```python
from build123d import *

# Parameters (mm, degrees)
SKETCH_1_W          = 103.9
SKETCH_1_H          = 75.8
EXTRUDE_1_DEPTH     = 5.7
SKETCH_2_R          = 3
SKETCH_2_R_2        = 1.65
SKETCH_2_W          = 5
SKETCH_2_H          = 4
SKETCH_2_R_3        = 1.15
SKETCH_2_W_2        = 9
EXTRUDE_2_DEPTH     = 2.5
FILLET_1_R          = 1
SKETCH_3_R          = 2.5
CUT_EXTRUDE_1_DEPTH = 1
SKETCH_4_W          = 95.04
SKETCH_4_H          = 53.86
CUT_EXTRUDE_2_DEPTH = 3


with BuildPart() as part:
    # 草图1 → 凸台-拉伸1 (new body)
    with BuildSketch(Plane(origin=(0, 0, 0), x_dir=(1, 0, 0), z_dir=(0, 1, 0))):
        Rectangle(SKETCH_1_W, SKETCH_1_H)
    extrude(amount=EXTRUDE_1_DEPTH)

    # 草图2 → 凸台-拉伸2 (add)
    # profile 1 of 12: a face of its own
    with BuildSketch(Plane(origin=(0, 0, 0), x_dir=(1, 0, 0), z_dir=(0, 1, 0))):
        with BuildLine():
            ThreePointArc((-53.4, 20.95), (-54.278679656, 18.828679656), (-56.4, 17.95))
            Line((-56.4, 17.95), (-51.95, 17.95))
            Line((-51.95, 17.95), (-51.95, 23.95))
            Line((-51.95, 23.95), (-56.4, 23.95))
            ThreePointArc((-56.4, 23.95), (-54.278679656, 23.071320344), (-53.4, 20.95))
        make_face()
    # profile 2 of 12: a face of its own
    with BuildSketch(Plane(origin=(0, 0, 0), x_dir=(1, 0, 0), z_dir=(0, 1, 0))):
        with Locations((-56.4, 20.95)):
            Circle(SKETCH_2_R)
        with Locations(Location((-56.4, 20.95, 0), (0, 0, 270))):
            Circle(SKETCH_2_R_2, mode=Mode.SUBTRACT)
    # profile 3 of 12: a face of its own
    with BuildSketch(Plane(origin=(0, 0, 0), x_dir=(1, 0, 0), z_dir=(0, 1, 0))):
        with Locations((-24.55, 39.9)):
            Rectangle(SKETCH_2_W, SKETCH_2_H)
        with Locations(Location((-24.55, 39.9, 0), (0, 0, 270))):
            Circle(SKETCH_2_R_3, mode=Mode.SUBTRACT)
    # profile 4 of 12: a face of its own
    with BuildSketch(Plane(origin=(0, 0, 0), x_dir=(1, 0, 0), z_dir=(0, 1, 0))):
        with Locations((24.55, 39.9)):
            Rectangle(SKETCH_2_W, SKETCH_2_H)
        with Locations(Location((24.55, 39.9, 0), (0, 0, 270))):
            Circle(SKETCH_2_R_3, mode=Mode.SUBTRACT)
    # profile 5 of 12: a face of its own
    with BuildSketch(Plane(origin=(0, 0, 0), x_dir=(1, 0, 0), z_dir=(0, 1, 0))):
        with BuildLine():
            Line((51.95, 17.95), (56.4, 17.95))
            ThreePointArc((56.4, 17.95), (53.4, 20.95), (56.4, 23.95))
            Line((56.4, 23.95), (51.95, 23.95))
            Line((51.95, 23.95), (51.95, 17.95))
        make_face()
    # profile 6 of 12: a face of its own
    with BuildSketch(Plane(origin=(0, 0, 0), x_dir=(1, 0, 0), z_dir=(0, 1, 0))):
        with Locations((56.4, 20.95)):
            Circle(SKETCH_2_R)
        with Locations(Location((56.4, 20.95, 0), (0, 0, 270))):
            Circle(SKETCH_2_R_2, mode=Mode.SUBTRACT)
    # profile 7 of 12: a face of its own
    with BuildSketch(Plane(origin=(0, 0, 0), x_dir=(1, 0, 0), z_dir=(0, 1, 0))):
        with Locations((56.4, -20.95)):
            Circle(SKETCH_2_R)
        with Locations(Location((56.4, -20.95, 0), (0, 0, 270))):
            Circle(SKETCH_2_R_2, mode=Mode.SUBTRACT)
    # profile 8 of 12: a face of its own
    with BuildSketch(Plane(origin=(0, 0, 0), x_dir=(1, 0, 0), z_dir=(0, 1, 0))):
        with BuildLine():
            ThreePointArc((56.4, -23.95), (53.4, -20.95), (56.4, -17.95))
            Line((56.4, -17.95), (51.95, -17.95))
            Line((51.95, -17.95), (51.95, -23.95))
            Line((51.95, -23.95), (56.4, -23.95))
        make_face()
    # profile 9 of 12: a face of its own
    with BuildSketch(Plane(origin=(0, 0, 0), x_dir=(1, 0, 0), z_dir=(0, 1, 0))):
        with Locations((34.9, -39.9)):
            Rectangle(SKETCH_2_W_2, SKETCH_2_H)
        with Locations(Location((37.4, -39.9, 0), (0, 0, 270))):
            Circle(SKETCH_2_R_3, mode=Mode.SUBTRACT)
        with Locations(Location((32.4, -39.9, 0), (0, 0, 270))):
            Circle(SKETCH_2_R_3, mode=Mode.SUBTRACT)
    # profile 10 of 12: a face of its own
    with BuildSketch(Plane(origin=(0, 0, 0), x_dir=(1, 0, 0), z_dir=(0, 1, 0))):
        with Locations((-35.5, -39.9)):
            Rectangle(SKETCH_2_W, SKETCH_2_H)
        with Locations(Location((-35.5, -39.9, 0), (0, 0, 270))):
            Circle(SKETCH_2_R_3, mode=Mode.SUBTRACT)
    # profile 11 of 12: a face of its own
    with BuildSketch(Plane(origin=(0, 0, 0), x_dir=(1, 0, 0), z_dir=(0, 1, 0))):
        with Locations((-56.4, -20.95)):
            Circle(SKETCH_2_R)
        with Locations(Location((-56.4, -20.95, 0), (0, 0, 270))):
            Circle(SKETCH_2_R_2, mode=Mode.SUBTRACT)
    # profile 12 of 12: a face of its own
    with BuildSketch(Plane(origin=(0, 0, 0), x_dir=(1, 0, 0), z_dir=(0, 1, 0))):
        with BuildLine():
            ThreePointArc((-53.4, -20.95), (-54.278679656, -23.071320344), (-56.4, -23.95))
            Line((-56.4, -23.95), (-51.95, -23.95))
            Line((-51.95, -23.95), (-51.95, -17.95))
            Line((-51.95, -17.95), (-56.4, -17.95))
            ThreePointArc((-56.4, -17.95), (-54.278679656, -18.828679656), (-53.4, -20.95))
        make_face()
    extrude(amount=EXTRUDE_2_DEPTH)

    # 圆角1
    fillet_1_edges = [part.edges().sort_by_distance(p)[0] for p in [
        (-27.05, 1.25, -41.9),
        (-22.05, 1.25, -41.9),
        (22.05, 1.25, -41.9),
        (27.05, 1.25, -41.9),
        (30.4, 1.25, 41.9),
        (39.4, 1.25, 41.9),
        (-38, 1.25, 41.9),
        (-33, 1.25, 41.9),
    ]]
    fillet(fillet_1_edges, radius=FILLET_1_R)

    # 草图3 → 切除-拉伸1 (cut)
    with BuildSketch(Plane(origin=(0, 2.5, 0), x_dir=(1, 0, 0), z_dir=(0, 1, 0))):
        with Locations(Location((-56.4, -20.95, 0), (0, 0, 270))):
            Circle(SKETCH_3_R)
        with Locations(Location((-56.4, 20.95, 0), (0, 0, 270))):
            Circle(SKETCH_3_R)
        with Locations(Location((56.4, 20.95, 0), (0, 0, 270))):
            Circle(SKETCH_3_R)
        with Locations(Location((56.4, -20.95, 0), (0, 0, 270))):
            Circle(SKETCH_3_R)
    extrude(amount=-CUT_EXTRUDE_1_DEPTH, mode=Mode.SUBTRACT)

    # 草图4 → 切除-拉伸2 (cut)
    with BuildSketch(Plane(origin=(0, 5.7, 0), x_dir=(1, 0, 0), z_dir=(0, 1, 0))):
        Rectangle(SKETCH_4_W, SKETCH_4_H)
    extrude(amount=-CUT_EXTRUDE_2_DEPTH, mode=Mode.SUBTRACT)


solid = part.part
```
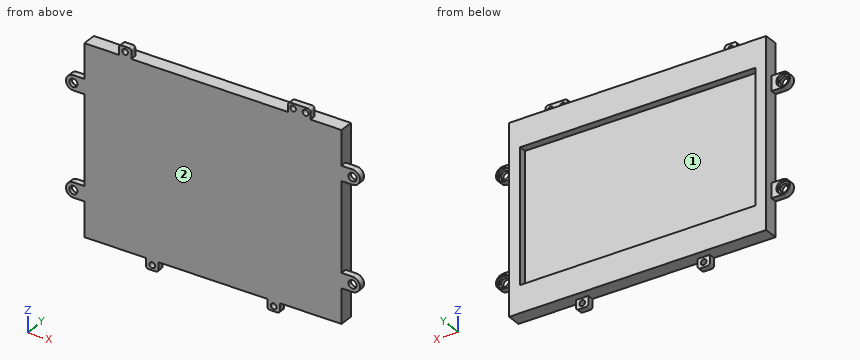
The listing builds one solid part. Answer for the finished solid, in the listing's coordinates (mm). Face numbers are marked on the shaded views. Coordinates: 2 decimals unless noted, no trailing zeros. Loops run counter-clockwise (first coordinate to the right, second up) from the corner with the lowest first, then second, coordinate; pieces in that order, holes last. Notation, with made-up numbers: M 79,51 L 114,51 A28 cw 114,69 Z; hole C -31,83.5 d6. An arc over 180 degrees is marked long. Answer as CSV lines item,"result". Start each with the question number.
(1) The part is cut by section D-D (z = -9.5). Give the vertices of the cut face in (x, y).
(2) Given pin 1 (1.5 mm diameter, centred on x = 56, z = -20, fed in from +Y); pin 2 (1.2 mm diameter, centred on y = 1, z = 39, fed in from -X); pin 3 (3 mm diameter, centred on y = 0.5, z = -38.5, fed in from -X), each flat-ended and moving along its own axis, determine where each tip first touches the part or whether it passes through.
(3) The part is cut by section B-B (z = -20.95). Give the vertices of the cut face in (x, y).
(4) Find the intervals of material crossed by L1, parallel to X at y = 0.85, z = 20.95; L2, parallel to Z at x = -56.4, y = 0.4; L3, parallel to X at y = 1.2, z = -39.9, in increasing order. Write a range as [from, to].
(5) The mould has two halves that part along X. Classify the marked faces 1 and 2: pulls with the +X half, pulls with the -X half, needs draft (parallel to the pull), parting line crosses it, or undercut.
(6) The part is cut by section A-A (y = 4). Give the vertices of the cut face in (x, z), and give its area (3 significant figures).
(7) The part is cut by section C-C (x = 11). Give the vertices of the cut face in (y, z), and give its area (3 significant figures).
Determined:
1,outline,"M -51.95,0 L 51.95,0 L 51.95,5.7 L 47.52,5.7 L 47.52,2.7 L -47.52,2.7 L -47.52,5.7 L -51.95,5.7 Z"
2,pin 1,"y = 1.5"
2,pin 2,"x = -38"
2,pin 3,"x = -51.95"
3,outline,"M -59.4,0 L -58.05,0 L -58.05,1.5 L -58.9,1.5 L -58.9,2.5 L -59.4,2.5 Z; M -54.75,0 L 54.75,0 L 54.75,1.5 L 53.9,1.5 L 53.9,2.5 L 51.95,2.5 L 51.95,5.7 L 47.52,5.7 L 47.52,2.7 L -47.52,2.7 L -47.52,5.7 L -51.95,5.7 L -51.95,2.5 L -53.9,2.5 L -53.9,1.5 L -54.75,1.5 Z; M 58.05,0 L 59.4,0 L 59.4,2.5 L 58.9,2.5 L 58.9,1.5 L 58.05,1.5 Z"
4,L1,"[-59.4, -58.05], [-54.75, 54.75], [58.05, 59.4]"
4,L2,"[-23.95, -22.6], [-19.3, -17.95], [17.95, 19.3], [22.6, 23.95]"
4,L3,"[-27.05, -25.7], [-23.4, -22.05], [22.05, 23.4], [25.7, 27.05]"
5,face 1,"undercut"
5,face 2,"needs draft"
6,outline,"M -51.95,-37.9 L 51.95,-37.9 L 51.95,37.9 L -51.95,37.9 Z; hole M -47.52,-26.93 L 47.52,-26.93 L 47.52,26.93 L -47.52,26.93 Z"
6,area,"2,760 mm2"
7,outline,"M 0,-37.9 L 5.7,-37.9 L 5.7,-26.93 L 2.7,-26.93 L 2.7,26.93 L 5.7,26.93 L 5.7,37.9 L 0,37.9 Z"
7,area,"270 mm2"
